Could you check a few things on this model? Use its own coordinates, in mm. Round coordinates to 2 decimals unless told otherwise and drop trailing zeros. Loops run counter-clockwise (first coordinate to the right, second up) from the corner with the lowest first, then second, coordinate; pieces in that order, holes last. Notation, with made-up numbers: M 65.5,-17 L 98.5,-17 A32 cw 98.5,11 Z; hole C -22.75,86.25 d3. An arc over 180 degrees is marked long. One line per item, written item: value. Start each with the question number.
Q1. Imagine slicing it at C-C (z = 3). Give the number of separate pieces and of enclosed holes in the cut face, then the cut area to 3 significant figures.
Q2. Please list where these lines run through material, in increasing order: line 1 along Y through (x, z) = (-15.5, 1.55) (3 decimals); line 2 along Y through (x, z) = (76, 2.15) (3 decimals); line 3 along Y through (x, z) = (18, 0.55).
Q3. Imagine slicing it at A-A (x = -44). Please give me the cut outline in (y, z) (3 decimals).
Q4. Imagine slicing it at D-D (x = 150.5). Please give me the cut outline in (y, z), then the cut area to 3 significant figures.
Q5. I'm going to push flat-ended pins straight in: pin 1 Ø13 at (x, y) = (0, 26.665) entering from -Z; pin 2 Ø1 at (x, z) = (118, 3) entering from +Y. Where does each tip first touch, or does it pass through?
Q6. Imagine slicing it at B-B (y = 64.5). Please give me the cut outline in (x, z), then the cut area to 3 significant figures.
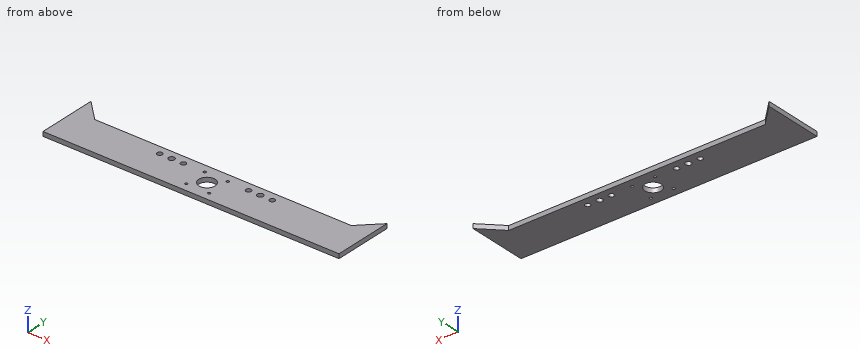
from build123d import *

# Parameters (mm, degrees)
BOSS_EXTRUDE1_DEPTH = 6
SKETCH2_R           = 11
SKETCH2_R_2         = 1.75
SKETCH2_R_3         = 4
SKETCH2_R_4         = 3.5
CUT_EXTRUDE1_DEPTH  = 216.490138986


with BuildPart() as part:
    # Sketch1 → Boss-Extrude1 (new body)
    with BuildSketch(Plane.XY):
        Polygon((-200, 0), (200, 0), (200, 80), (173.333333333, 53.333333333), (-173.333333333, 53.333333333), (-200, 80), align=None)
    extrude(amount=BOSS_EXTRUDE1_DEPTH)

    # Sketch2 → Cut-Extrude1 (cut, through all)
    with BuildSketch(Plane.XY.offset(6)):
        with Locations((0, 26.665)):
            Circle(SKETCH2_R)
        with Locations((15.5, 42.165)):
            Circle(SKETCH2_R_2)
        with Locations(Location((-15.5, 42.165, 0), (0, 0, 180))):
            Circle(SKETCH2_R_2)
        with Locations((-15.5, 11.165)):
            Circle(SKETCH2_R_2)
        with Locations(Location((15.5, 11.165, 0), (0, 0, 180))):
            Circle(SKETCH2_R_2)
        with Locations((60, 41.665)):
            Circle(SKETCH2_R_3)
        with Locations((76, 41.665)):
            Circle(SKETCH2_R_4)
        with Locations((44, 41.665)):
            Circle(SKETCH2_R_4)
        with Locations(Location((-44, 41.665, 0), (0, 0, 180))):
            Circle(SKETCH2_R_4)
        with Locations(Location((-76, 41.665, 0), (0, 0, 180))):
            Circle(SKETCH2_R_4)
        with Locations(Location((-60, 41.665, 0), (0, 0, 180))):
            Circle(SKETCH2_R_3)
    extrude(amount=-CUT_EXTRUDE1_DEPTH, mode=Mode.SUBTRACT)


solid = part.part
Report:
1. separate pieces: 1
1. enclosed holes: 11
1. area: 21,400 mm²
2. line 1: y = 0 to 9.415, 12.915 to 40.415, 43.915 to 53.333
2. line 2: y = 0 to 38.165, 45.165 to 53.333
2. line 3: y = 0 to 53.33
3. outline: M 0,0 L 38.165,0 L 38.165,6 L 0,6 Z; M 45.165,0 L 53.333,0 L 53.333,6 L 45.165,6 Z
4. outline: M 0,0 L 53.33,0 L 53.33,6 L 0,6 Z
4. area: 320 mm²
5. pin 1: passes through
5. pin 2: stops at y = 53.33
6. outline: M -200,0 L -184.5,0 L -184.5,6 L -200,6 Z; M 184.5,0 L 200,0 L 200,6 L 184.5,6 Z
6. area: 186 mm²
